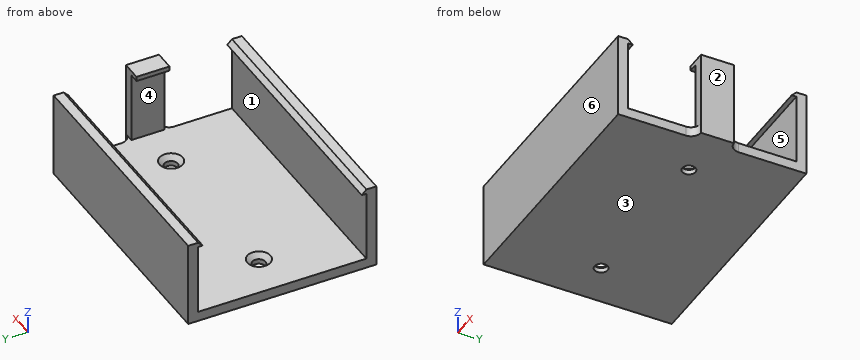
```python
from build123d import *

# Parameters (mm, degrees)
F1_DEPTH        = 38.3
F2_W            = 76.6
F2_H            = 51
F3_DEPTH        = 19.6
F5_DEPTH        = 76.6
F7_DEPTH        = 3
F8_W            = 10
F8_H            = 21.6
F9_DEPTH        = 3
F10_R           = 2.99999
F12_D           = 4
F12_CSINK_D     = 7
F12_CSINK_ANGLE = 90


# Not quite as in the source:
# - a fillet or chamfer is up to 0.001 mm smaller than in the source, because OpenCascade refuses the exact size


with BuildPart() as f1:
    # F0 (on Right) → F1 (new body, symmetric)
    with BuildSketch(Plane.YZ):
        Polygon((-28.5, 13), (-28.5, -13), (-5, -13), (0, -13), (5, -13), (28.5, -13), (28.5, 13), (5, 13), (-5, 13), align=None)
        Polygon((-5, -10), (-25.5, -10), (-25.5, 10), (-5, 10), (5, 10), (25.5, 10), (25.5, -10), (5, -10), align=None, mode=Mode.SUBTRACT)
    extrude(amount=F1_DEPTH, both=True)

    # F2 (on face) → F3 (cut)
    with BuildSketch(Plane.XY.offset(13)):
        Rectangle(F2_W, F2_H)
    extrude(amount=-F3_DEPTH, mode=Mode.SUBTRACT)

    # F4 (on face) → F5 (join)
    with BuildSketch(Plane.YZ.offset(38.3)):
        Polygon((24.0857864376, 11.5857864376), (25.5, 11.5857864376), (25.5, 13), align=None)
        Polygon((-24.0857864376, 11.5857864376), (-25.5, 13), (-25.5, 11.5857864376), align=None)
    extrude(amount=-F5_DEPTH)

    # F6 (on face) → F7 (join, symmetric)
    with BuildSketch(Plane.YZ.offset(38.3)):
        Polygon((-5, -13), (0, -13), (5, -13), (5, 13), (-5, 13), align=None)
    extrude(amount=F7_DEPTH, both=True)

    # F8 (on face) → F9 (cut)
    with BuildSketch(Plane(origin=(35.3, 0, 0), x_dir=(0, -1, 0), z_dir=(-1, 0, 0))):
        with Locations((0, 0.8)):
            Rectangle(F8_W, F8_H)
    extrude(amount=-F9_DEPTH, mode=Mode.SUBTRACT)

    # F10 (radius 3 in the source; OpenCascade refuses exactly that, so slightly less here)
    f10_edges = [f1.edges().sort_by_distance(p)[0] for p in [
        (38.3, -5, -11.5),
        (38.3, 5, -11.5),
    ]]
    fillet(f10_edges, radius=F10_R)

    # F12 (through all)
    with Locations(Plane.XY.offset(-10)):
        with Locations((-25, 0), (25, 0)):
            CounterSinkHole(F12_D / 2, F12_CSINK_D / 2, counter_sink_angle=F12_CSINK_ANGLE)


solid = f1.part
```
CAD build for the part. Positions are in the model's coordinates, mm. Face numbers are marked on the shaded views. A direction names the side the tool comes from. Give positions to 0.01 mm unless a question says otherwise; leave off trailing zeros. Order: outer loops, then holes, each group sorted by start corner. A loop starts at its lowest first (then second) coordinate and runs counter-clockwise, first axis right, second up.
(1) Mould opens along Z. For the marked faces 1, 2 and 3 say: released by +Z, released by -Z, zero draft, split by the parting line, or undercut.
(2) Drill centre lines: L1, parallel to X at y = 0, z = -12.15; L2, parallel to Y at x = 29, z = -7.75; L3, parallel to Y at x = 25, z = -12.5. Where is each one in solid material? Low to high.
(3) Tool access for the marked faces 4, 5 and 6: list every direction of +Z, -Z, +X, -X, +Y, -Y with a clear straight run to the whole face (end or side of a thin tool).
(4) Saw through at B-B, the plane z = 10. Give the cut face in (x, y), then the cut area to 3 significant figures.
(5) Flat gauge pins, fed straight in: pin 1 (3 mm diameter, centred on x = 39.5, z = 4.5, fed in from +Y); pin 2 (3 mm diameter, centred on y = 0, z = -2.5, fed in from -X); pin 3 (15.5 mm diameter, centred on x = 14, y = 1.5, fed in from +Z); pin 4 (1.1 mm diameter, centred on y = 2, z = 12.5, fed in from -X). Where does each tip first touch, or does it go through?
(6) Saw through at C-C, the plane y = 0. Give the cut face in (x, z), then the cut area to 4 significant figures.
(7) Saw through at A-A, the plane x = 25. Give the cut face in (y, z), then the cut area to 3 significant figures.
(8) Saw through at D-D, the plane x = -1.5. Give the cut face in (y, z), then the cut area to 3 significant figures.
Results found:
1. face 1: undercut
1. face 2: zero draft
1. face 3: released by -Z
2. L1: x = -38.3 to -27, -23 to 23, 27 to 41.3
2. L2: y = -28.5 to -25.5, 25.5 to 28.5
2. L3: y = -28.5 to -2, 2 to 28.5
3. face 4: -X
3. face 5: +X, -X
3. face 6: +Z, -Z, +X, -X, -Y
4. outline: (-38.3, -28.5) - (38.3, -28.5) - (38.3, -25.5) - (-38.3, -25.5) - close; (-38.3, 25.5) - (38.3, 25.5) - (38.3, 28.5) - (-38.3, 28.5) - close; (38.3, -5) - (41.3, -5) - (41.3, 5) - (38.3, 5) - close
4. area: 490 mm2
5. pin 1: stops at y = 28.5
5. pin 2: stops at x = 38.3
5. pin 3: stops at z = -10
5. pin 4: stops at x = 35.3
6. outline: (-38.3, -13) - (-27, -13) - (-27, -11.5) - (-28.5, -10) - (-38.3, -10) - close; (-23, -13) - (23, -13) - (23, -11.5) - (21.5, -10) - (-21.5, -10) - (-23, -11.5) - close; (27, -13) - (41.3, -13) - (41.3, 13) - (35.3, 13) - (35.3, 11.6) - (38.3, 11.6) - (38.3, -10) - (28.5, -10) - (27, -11.5) - close
6. area: 283.5 mm2
7. outline: (-28.5, -13) - (-2, -13) - (-2, -11.5) - (-3.5, -10) - (-25.5, -10) - (-25.5, 11.59) - (-24.09, 11.59) - (-25.5, 13) - (-28.5, 13) - close; (2, -13) - (28.5, -13) - (28.5, 13) - (25.5, 13) - (24.09, 11.59) - (25.5, 11.59) - (25.5, -10) - (3.5, -10) - (2, -11.5) - close
7. area: 297 mm2
8. outline: (-28.5, -13) - (28.5, -13) - (28.5, 13) - (25.5, 13) - (24.09, 11.59) - (25.5, 11.59) - (25.5, -10) - (-25.5, -10) - (-25.5, 11.59) - (-24.09, 11.59) - (-25.5, 13) - (-28.5, 13) - close
8. area: 311 mm2
